from build123d import *

# Parameters (mm, degrees)
ESQUISSE1_R             = 16
BOSS_EXTRU_1_DEPTH      = 35
ESQUISSE2_R             = 12.5
BOSS_EXTRU_2_DEPTH      = 55
ESQUISSE3_R             = 3
BOSS_EXTRU_3_DEPTH      = 15
ENL_V_START             = -15
ENL_V_MAT_EXTRU_1_DEPTH = 15
ESQUISSE5_R             = 10
BOSS_EXTRU_4_DEPTH      = 3
ESQUISSE8_R             = 1.5
ENL_V_MAT_EXTRU_2_DEPTH = 10
BOSS_EXTRU_5_DEPTH      = 20
ESQUISSE10_W            = 16.98090883
ESQUISSE10_H            = 7.182585406
ENL_V_MAT_EXTRU_3_DEPTH = 12
ESQUISSE12_W            = 1
ESQUISSE12_H            = 1
BOSS_EXTRU_6_DEPTH      = 12


with BuildPart() as part:
    # Esquisse1 → Boss.-Extru.1 (new body)
    with BuildSketch(Plane(origin=(0, 0, 0), x_dir=(1, 0, 0), z_dir=(0, 1, 0))):
        with Locations(Location((0, 0, 0), (0, 0, 270))):
            Circle(ESQUISSE1_R)
    extrude(amount=BOSS_EXTRU_1_DEPTH)

    # Esquisse2 → Boss.-Extru.2 (add)
    with BuildSketch(Plane.XZ):
        with Locations(Location((0, 0, 0), (0, 0, 270))):
            Circle(ESQUISSE2_R)
    extrude(amount=BOSS_EXTRU_2_DEPTH)

    # Esquisse3 → Boss.-Extru.3 (add)
    with BuildSketch(Plane(origin=(0, 35, 0), x_dir=(1, 0, 0), z_dir=(0, 1, 0))):
        with Locations(Location((0, 0, 0), (0, 0, 270))):
            Circle(ESQUISSE3_R)
    extrude(amount=BOSS_EXTRU_3_DEPTH)

    # Esquisse4 → Enlèv. mat.-Extru.1 (cut)
    with BuildSketch(Plane(origin=(0, 50, 0), x_dir=(1, 0, 0), z_dir=(0, 1, 0)).offset(ENL_V_START)):
        with BuildLine():
            Line((2.946395849, 0.56458082), (0, -3))
            ThreePointArc((0, -3), (2.31233026, -1.911315979), (2.946395849, 0.56458082))
        make_face()
    extrude(amount=ENL_V_MAT_EXTRU_1_DEPTH, mode=Mode.SUBTRACT)

    # Esquisse5 → Boss.-Extru.4 (add)
    with BuildSketch(Plane(origin=(0, 35, 0), x_dir=(1, 0, 0), z_dir=(0, 1, 0))):
        with Locations(Location((0, 0, 0), (0, 0, 270))):
            Circle(ESQUISSE5_R)
    extrude(amount=BOSS_EXTRU_4_DEPTH)

    # Esquisse8 → Enlèv. mat.-Extru.2 (cut)
    with BuildSketch(Plane(origin=(0, 35, 0), x_dir=(1, 0, 0), z_dir=(0, 1, 0))):
        with Locations(Location((-9.363786072, 9.017733108, 0), (0, 0, 270))):
            Circle(ESQUISSE8_R)
        with Locations(Location((9.363786072, 9.017733108, 0), (0, 0, 270))):
            Circle(ESQUISSE8_R)
        with Locations(Location((-9.363786072, -9.017733108, 0), (0, 0, 270))):
            Circle(ESQUISSE8_R)
        with Locations(Location((9.363786072, -9.017733108, 0), (0, 0, 270))):
            Circle(ESQUISSE8_R)
    extrude(amount=-ENL_V_MAT_EXTRU_2_DEPTH, mode=Mode.SUBTRACT)

    # Esquisse9 → Boss.-Extru.5 (add)
    with BuildSketch(Plane.XZ.offset(55)):
        with BuildLine():
            Line((0, 13.5), (-26.340367248, 13.5))
            Line((-26.340367248, 13.5), (-26.340367248, -13.5))
            Line((-26.340367248, -13.5), (0, -13.5))
            ThreePointArc((0, -13.5), (13.5, 0), (0, 13.5))
        make_face()
    extrude(amount=BOSS_EXTRU_5_DEPTH)

    # Esquisse10 → Enlèv. mat.-Extru.3 (cut)
    with BuildSketch(Plane.ZY.offset(26.340367248)):
        with Locations((0, -60.318042099)):
            Rectangle(ESQUISSE10_W, ESQUISSE10_H)
    extrude(amount=-ENL_V_MAT_EXTRU_3_DEPTH, mode=Mode.SUBTRACT)

    # Esquisse12 → Boss.-Extru.6 (add)
    with BuildSketch(Plane.ZY.offset(14.340367248)):
        with Locations((-1.990454415, -58.574860414)):
            Rectangle(ESQUISSE12_W, ESQUISSE12_H)
        with Locations((-3.990454415, -58.574860414)):
            Rectangle(ESQUISSE12_W, ESQUISSE12_H)
        with Locations((0.009545585, -58.574860414)):
            Rectangle(ESQUISSE12_W, ESQUISSE12_H)
        with Locations((2.009545585, -58.574860414)):
            Rectangle(ESQUISSE12_W, ESQUISSE12_H)
        with Locations((4.009545585, -58.574860414)):
            Rectangle(ESQUISSE12_W, ESQUISSE12_H)
    extrude(amount=BOSS_EXTRU_6_DEPTH)


solid = part.part
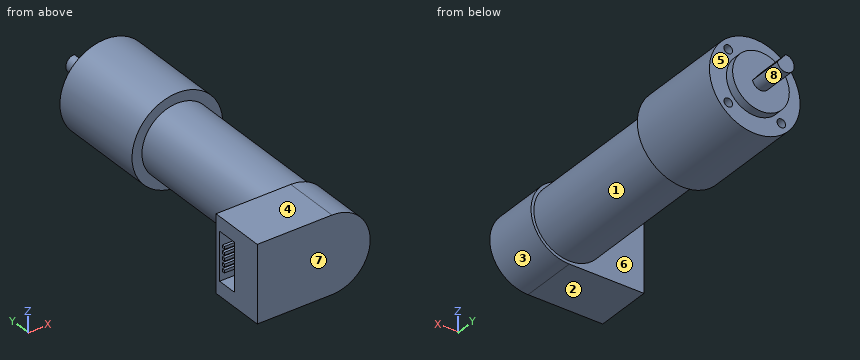
The listing builds one solid part. Answer for the finished solid, in the listing's coordinates (mm). Face numbers are marked on the shaded views. A direction names the side the tool comes from. Round coordinates to 2 decimals unless told otherwise and drop trailing zeros. Order: outer loops, then holes, each group sorted by start corner. A loop starts at its lowest first (then second) coordinate and runs counter-clockwise, first axis right, second up. Notation, with made-up numbers: (72, 15) -> (99, 15) arc R24 cw to (99, 43) -> close; hole circle Ø6 at (76, 23). An arc over 180 degrees is marked (long way). Write each question's results on one line, items separated by ' | '. Start each with the question number.
Q1. Which of the six approach directions +Z, -Z, +X, -X, +Y, -Y give full straight-line access (tool end or side, diameter ignored) to the marked faces 1, 2, 3, 4 and 5?
Q2. Each of these flat-tipped pins is pushed along its axis until it touches: pin 1 (12 mm diameter, centred on y = -25.5, z = -0.5, fed in from +X); pin 2 (1.5 mm diameter, centred on y = -30, z = -3, fed in from +X); pin 3 (3 mm diameter, centred on x = -0.5, y = -17, fed in from -Z). Where does it stop, or does it pass through?
Q3. The mould has two halves that part along Y. Classify the marked faces 6, 7 and 8: pulls with the +Y half, pulls with the -Y half, needs draft (parallel to the pull), parting line crosses it, or undercut.
Q4. Straight lines are drawn through the part: probe 1 along Y at (x, z) = (-22, 5); probe 2 along Y at (x, z) = (-5, 12); probe 3 along Y at (x, z) = (-11.5, 12). For each, find the intervals that lie inside material, in ascending order. Write a range as from..to.
Q5. Find section B-B (z = -6). Determine the outline of the cut face in (x, y), then the cut area to 4 significant figures.
Q6. Find section A-A (x = -20). Determine the outline of the cut face in (y, z).
Q7. Find section C-C (y = -38). Determine the outline of the cut face in (x, z), then the cut area to 3 significant figures.
Worked answers:
1) face 1: none | face 2: -Z, +X, -X, -Y | face 3: +X, -Y | face 4: +Z, +X, -X, -Y | face 5: +Y
2) pin 1: stops at x = 12.5 | pin 2: stops at x = 12.3 | pin 3: stops at z = -12.5
3) face 6: undercut | face 7: pulls with the -Y half | face 8: needs draft
4) probe 1: y = -75..-63.91, -56.73..-55 | probe 2: y = -75..-55, 0..35 | probe 3: y = -75..-55
5) outline: (-26.34, -75) -> (12.09, -75) -> (12.09, -55) -> (10.97, -55) -> (10.97, 0) -> (14.83, 0) -> (14.83, 35) -> (8, 35) -> (8, 38) -> (-8, 38) -> (-8, 35) -> (-14.83, 35) -> (-14.83, 0) -> (-10.97, 0) -> (-10.97, -55) -> (-26.34, -55) -> (-26.34, -56.73) -> (-14.34, -56.73) -> (-14.34, -63.91) -> (-26.34, -63.91) -> close | area: 2,975 mm2
6) outline: (-75, -13.5) -> (-55, -13.5) -> (-55, 13.5) -> (-75, 13.5) -> close; (-59.07, -4.49) -> (-58.07, -4.49) -> (-58.07, -3.49) -> (-59.07, -3.49) -> close; (-59.07, -2.49) -> (-58.07, -2.49) -> (-58.07, -1.49) -> (-59.07, -1.49) -> close; (-59.07, -0.49) -> (-58.07, -0.49) -> (-58.07, 0.51) -> (-59.07, 0.51) -> close; (-59.07, 1.51) -> (-58.07, 1.51) -> (-58.07, 2.51) -> (-59.07, 2.51) -> close; (-59.07, 3.51) -> (-58.07, 3.51) -> (-58.07, 4.51) -> (-59.07, 4.51) -> close; hole (-63.91, -8.49) -> (-56.73, -8.49) -> (-56.73, 8.49) -> (-63.91, 8.49) -> close
7) outline: circle Ø25 at (0, 0) | area: 491 mm2
